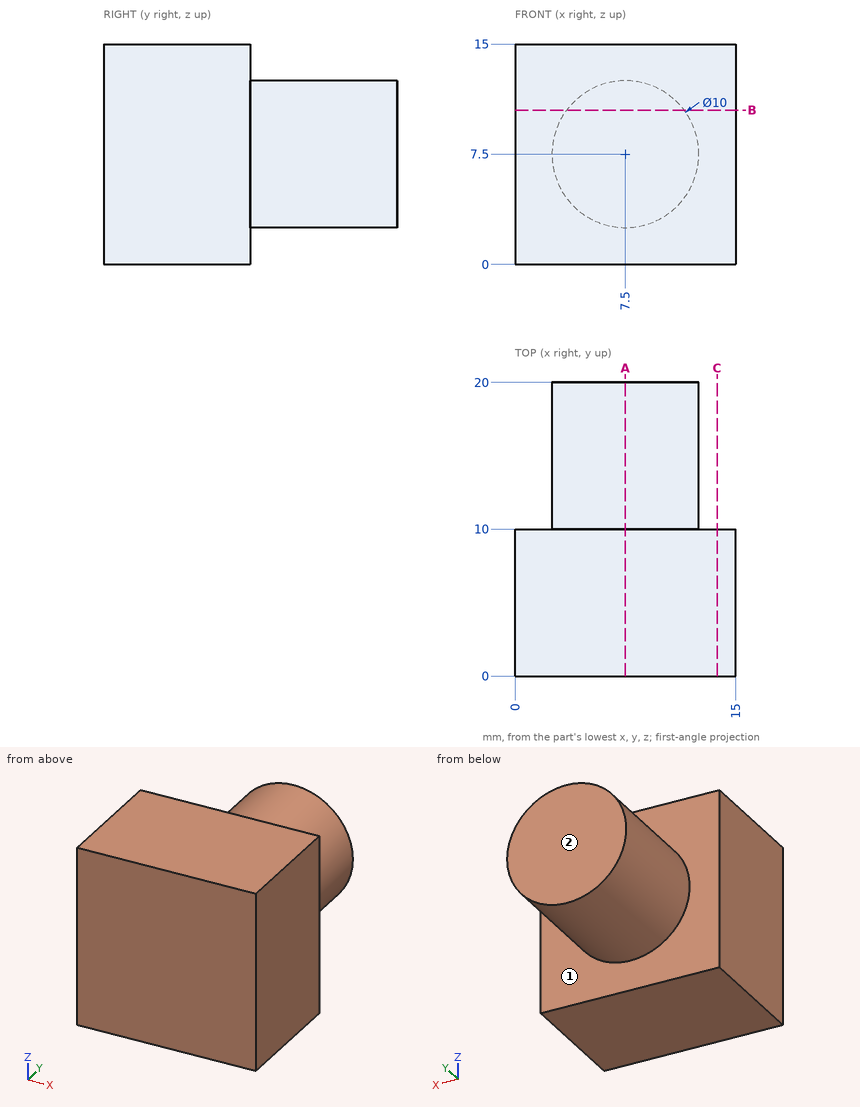
Geometry: see drawing. Coordinates: mm, zero at the bounding-box minimum. A direction names the side the tool comes from. Round coordinates to 2 decimals unless told otherwise and drop trailing zeros. Loops run counter-clockwise (first coordinate to the right, second up) from the corner with the lowest first, then second, coordinate; pieces in that order, holes last. Notation, with made-up numbers: (-37.5, 27.5) - (-12.5, 27.5) arc R24 ccw to (-12.5, 63.5) - close; hole circle Ø3 at (-22.75, -39). An arc over 180 degrees is marked (long way). Write item = value, one per line. Start each with the question number.
(1) Pin query (flat end, axial travel): pin 1 (4 mm diameter, centred on x = 7, y = 18, fed in from -Z); pin 2 (1.5 mm diameter, centred on x = 9.5, y = 15, fed in from +Z); pin 3 (1.5 mm diameter, centred on y = 14.5, z = 9, fed in from -X). Return the tip coordinate at first contact, or that it passes through.
(2) Section query A-A, the plane x = 7.5. Output: boundary loops of the cut face in (y, z).
(3) Section query B-B, the plane z = 10.5. Output: boundary loops of the cut face in (x, y), plus the area to 3 significant figures.
(4) Ray query, line 1 along Z through (x, y) = (7.25, 13.5); line 2 along Y through (x, z) = (2, 7); line 3 along X through (y, z) = (12.5, 6.25). Return the intervals inside material, ascending. Write a range as from..to.
(5) Set-up query: the marked faces 1 and 2. Return all of +Z, -Z, +X, -X, +Y, -Y with unobstructed straight access to the full face (end or side cutting, diameter ignored); none if empty.
(6) Section query C-C, the plane x = 13.75. Output: boundary loops of the cut face in (y, z).
Conclusion:
q1.pin_1 = 2.5
q1.pin_2 = 12.34
q1.pin_3 = 2.56
q2.outline = (0, 0) - (10, 0) - (10, 2.5) - (20, 2.5) - (20, 12.5) - (10, 12.5) - (10, 15) - (0, 15) - close
q3.outline = (0, 0) - (15, 0) - (15, 10) - (11.5, 10) - (11.5, 20) - (3.5, 20) - (3.5, 10) - (0, 10) - close
q3.area = 230 mm2
q4.line_1 = 2.51..12.49
q4.line_2 = 0..10
q4.line_3 = 2.66..12.34
q5.face_1 = +Y
q5.face_2 = +Z, -Z, +X, -X, +Y
q6.outline = (0, 0) - (10, 0) - (10, 15) - (0, 15) - close
